Check sheet for the modelled part. Datum: model origin and axes. Units: mm. A direction names the side the tool comes from. Coordinates: 2 decimals unless noted, no trailing zeros. Loops run counter-clockwise (first coordinate to the right, second up) from the corner with the lowest first, then second, coordinate; pieces in that order, holes last. Notation, with made-up numbers: (17, -28) - (66, -28) arc R25 cw to (66, 8) - close; hole circle Ø8 at (-25, -24). An arc over 180 degrees is marked (long way). Use a Markdown table: item, result. Add a question column.
1) Tool access check on faces 4 (the flat face through (0, 3, 0)), 5 (the cylindrical face through (-0.55, -2.48, 84.52)). Record the directions out of +Z, -Z, +X, -X, +Y, -Y that give a thin tool (end or side, any length) a straight path to the whole face; none if there is none.
2) Sectioned sample at C-C, the plane z = 156.5. Enter the section's corners in (x, y) (3 decimals), then the cut area to 3 significant figures.
3) Draft check along X on faces 1 (the flat face through (0, 0, 172.085)), 2 (the flat face through (0, 0, 171.45)), 3 (the cylindrical face through (-0.69, -3.1, 84.84)). Enter one of: pulls with the +X half, pulls with the -X half, needs draft (parallel to the pull), parting line crosses it, or undercut.
4) Sectioned sample at B-B, the plane y = 0. Enter the section's corners in (x, z) (3 decimals).
5) Thickness scan on line 1 (Y direction, x = 0, z = 124.5) (3 decimals); line 2 (X direction, y = -0.25, z = 33.5); line 3 (X direction, y = -1, z = 92). Record the ranges inside material, lowest first.
6) Go/stop test with flat-tipped pins: P1, Ø1.5, axis at y = 1, z = 128, coming from the -X side; P2, Ø1.5, axis at x = 0.5, y = -0.5, coming from the -Z side. Record where each tip stops, or that it passes through.
from build123d import *

# Parameters (mm, degrees)
SKETCH1_R           = 3.175
BOSS_EXTRUDE1_DEPTH = 172.085
SHELL1_T            = -0.635
SKETCH3_R           = 1.27
CUT_EXTRUDE3_DEPTH  = 5.08


with BuildPart() as part:
    # Sketch1 → Boss-Extrude1 (new body)
    with BuildSketch(Plane.XY):
        Circle(SKETCH1_R)
    extrude(amount=BOSS_EXTRUDE1_DEPTH)

    # Shell1
    shell1_openings = [part.faces().sort_by_distance(p)[0] for p in [
        (0, 0, 0),
    ]]
    offset(amount=SHELL1_T, openings=shell1_openings, kind=Kind.INTERSECTION)

    # Sketch3 → Cut-Extrude3 (cut)
    with BuildSketch(Plane(origin=(0, 0, 0), x_dir=(1, 0, 0), z_dir=(0, 1, 0))):
        with Locations(Location((0, -83.5025, 0), (0, 0, 90))):
            Circle(SKETCH3_R)
    extrude(amount=CUT_EXTRUDE3_DEPTH, mode=Mode.SUBTRACT)


solid = part.part
Solved:
| question | item | result |
|---|---|---|
| 1 | face 4 | -Z, +X, -X, +Y, -Y |
| 1 | face 5 | -Z |
| 2 | outline | circle Ø6.35 at (0, 0); hole circle Ø5.08 at (0, 0) |
| 2 | area | 11.4 mm2 |
| 3 | face 1 | needs draft |
| 3 | face 2 | undercut |
| 3 | face 3 | parting line crosses it |
| 4 | outline | (-3.175, 0) - (-2.54, 0) - (-2.54, 171.45) - (2.54, 171.45) - (2.54, 0) - (3.175, 0) - (3.175, 172.085) - (-3.175, 172.085) - close |
| 5 | line 1 | y = -3.175 to -2.54, 2.54 to 3.175 |
| 5 | line 2 | x = -3.17 to -2.53, 2.53 to 3.17 |
| 5 | line 3 | x = -3.01 to -2.33, 2.33 to 3.01 |
| 6 | P1 | stops at x = -3.17 |
| 6 | P2 | stops at z = 171.45 |
